from build123d import *

# Parameters (mm, degrees)
SKETCH1_R           = 25.25
SKETCH1_R_2         = 12
BOSS_EXTRUDE1_DEPTH = 6
BOSS_EXTRUDE2_START = -5
SKETCH2_R           = 37
SKETCH2_R_2         = 12
BOSS_EXTRUDE2_DEPTH = 5
SKETCH3_R           = 1.5
CUT_EXTRUDE1_DEPTH  = 53.668776329
CUT_EXTRUDE2_START  = -3
SKETCH4_R           = 3.5
CUT_EXTRUDE2_DEPTH  = 56.668776329
CIRPATTERN1_COUNT   = 3
CHAMFER1_SIZE       = 12
CHAMFER1_SIZE_2     = 6.92820323
CHAMFER2_SIZE       = 2
SKETCH5_R           = 2.1
CUT_EXTRUDE3_DEPTH  = 54.46961768
CIRPATTERN2_COUNT   = 6
FILLET1_R           = 1


with BuildPart() as part:
    # Sketch1 → Boss-Extrude1 (new body)
    with BuildSketch(Plane(origin=(0, 0, 0), x_dir=(1, 0, 0), z_dir=(0, 1, 0))):
        with Locations(Location((0, 0, 0), (0, 0, 270))):
            Circle(SKETCH1_R)
        with Locations(Location((0, 0, 0), (0, 0, 270))):
            Circle(SKETCH1_R_2, mode=Mode.SUBTRACT)
    extrude(amount=BOSS_EXTRUDE1_DEPTH)

    # Sketch2 → Boss-Extrude2 (add)
    with BuildSketch(Plane(origin=(0, 0, 0), x_dir=(1, 0, 0), z_dir=(0, 1, 0)).offset(BOSS_EXTRUDE2_START)):
        with Locations(Location((0, 0, 0), (0, 0, 270))):
            Circle(SKETCH2_R)
        with Locations(Location((0, 0, 0), (0, 0, 270))):
            Circle(SKETCH2_R_2, mode=Mode.SUBTRACT)
    extrude(amount=BOSS_EXTRUDE2_DEPTH)

    # Sketch3 → Cut-Extrude1 (cut, through all)
    with BuildSketch(Plane(origin=(0, 0, 0), x_dir=(1, 0, 0), z_dir=(0, 1, 0))):
        with Locations(Location((0, 32, 0), (0, 0, 270))):
            Circle(SKETCH3_R)
    cut_extrude1 = extrude(amount=-CUT_EXTRUDE1_DEPTH, mode=Mode.SUBTRACT)

    # Sketch4 → Cut-Extrude2 (cut)
    with BuildSketch(Plane(origin=(0, 0, 0), x_dir=(1, 0, 0), z_dir=(0, 1, 0)).offset(CUT_EXTRUDE2_START)):
        with Locations(Location((0, 32, 0), (0, 0, 270))):
            Circle(SKETCH4_R)
    cut_extrude2 = extrude(amount=CUT_EXTRUDE2_DEPTH, mode=Mode.SUBTRACT)

    # CirPattern1: Cut-Extrude1, Cut-Extrude2 ×3 about axis
    cirpattern1_axis = Axis((0, 0, 0), (0, 1, 0))
    add([cut_extrude1.rotate(cirpattern1_axis, i * 360 / CIRPATTERN1_COUNT) for i in range(1, CIRPATTERN1_COUNT)], mode=Mode.SUBTRACT)
    add([cut_extrude2.rotate(cirpattern1_axis, i * 360 / CIRPATTERN1_COUNT) for i in range(1, CIRPATTERN1_COUNT)], mode=Mode.SUBTRACT)

    # Chamfer1
    # the kernel refuses this chamfer: 12, 6.92820323 mm, written as the material it takes off along each edge
    with BuildSketch(Plane(origin=(0, -5, 0), x_dir=(0, 0, 1), z_dir=(-1, 0, 0))) as chamfer1_piece_1:
        Polygon((12, CHAMFER1_SIZE), (12 + CHAMFER1_SIZE_2, 0), (12, 0), align=None)
    revolve(axis=Axis((0, -5, 0), (0, 1, 0)), mode=Mode.SUBTRACT)

    # Chamfer2
    # the kernel refuses this chamfer: 2 mm, written as the material it takes off along each edge
    with BuildSketch(Plane(origin=(0, 0, 0), x_dir=(0, 0, 1), z_dir=(-1, 0, 0))) as chamfer2_piece_1:
        Polygon((37 - CHAMFER2_SIZE, 0), (37, -CHAMFER2_SIZE), (37, 0), align=None)
    revolve(axis=Axis((0, 0, 0), (0, 1, 0)), mode=Mode.SUBTRACT)

    # Sketch5 → Cut-Extrude3 (cut, through all)
    with BuildSketch(Plane(origin=(0, 6, 0), x_dir=(1, 0, 0), z_dir=(0, 1, 0))):
        with Locations(Location((0, 16.5, 0), (0, 0, 270))):
            Circle(SKETCH5_R)
    cut_extrude3 = extrude(amount=-CUT_EXTRUDE3_DEPTH, mode=Mode.SUBTRACT)

    # CirPattern2: Cut-Extrude3 ×6 about axis
    cirpattern2_axis = Axis((0, 0, 0), (0, 1, 0))
    for i in range(1, CIRPATTERN2_COUNT):
        add(cut_extrude3.rotate(cirpattern2_axis, i * 360 / CIRPATTERN2_COUNT), mode=Mode.SUBTRACT)

    # Fillet1
    fillet1_edges = [part.edges().sort_by_distance(p)[0] for p in [
        (0, 6, -12.577350269),
    ]]
    fillet(fillet1_edges, radius=FILLET1_R)


solid = part.part
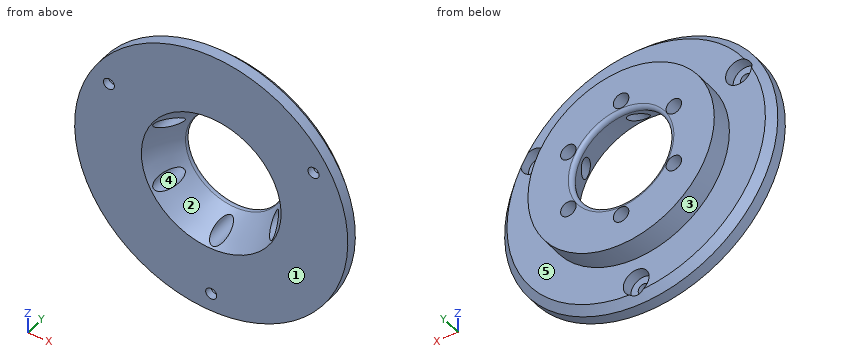
Source: CAD feature listing. Evaluate the final solid. Frame: model axes, mm. Face numbers are marked on the shaded views. A direction names the side the tool comes from. Give positions to 0.01 mm unless a question says otherwise; leave off trailing zeros. Write each loop counter-clockwise with the first axis right and the second up, starting at its lowest first coordinate (ties: lowest second). Pieces come first, ordered by that corner, then holes. Notation, with made-up numbers: (-13.75, -21.5) -> (9.25, -21.5) arc R14 ccw to (9.25, -17.5) -> close; hole circle Ø4 at (43.5, -35.75). An arc over 180 degrees is marked (long way). Write item = value, one per line.
Q1. Line query: line 1 (X direction, y = -4.1, z = 16); line 2 (Y direction, x = -24.5, z = 18.5); line 3 (Z direction, x = 11, y = 4). Output: solid intervals per line, ascending. Write a range as from..to.
Here are the results:
line_1 = -33.36..-29.21, -26.21..-9.1, 9.1..26.21, 29.21..33.36
line_2 = -5..0
line_3 = -22.73..-8.22, 8.22..22.73
Q2. Cut plane A-A on z = 0. Return loops of the section in (x, y), then the cut area to 3 significant figures.
Here are the results:
outline = (-37, -5) -> (-18.93, -5) -> (-13.44, 4.5) arc R1 ccw to (-14.31, 6) -> (-25.25, 6) -> (-25.25, 0) -> (-35, 0) -> (-37, -2) -> close; (13.44, 4.5) -> (18.93, -5) -> (37, -5) -> (37, -2) -> (35, 0) -> (25.25, 0) -> (25.25, 6) -> (14.31, 6) arc R1 ccw to start
area = 321 mm²
Q3. Cut plane B-B on y = 1.75. Return loops of the section in (x, z), then the cut area to 3 significant figures.
Here are the results:
outline = circle Ø50.5 at (0, 0); hole (-13.67, -6.24) arc R2.1 ccw (long way) to (-12.24, -8.72) arc R15.03 ccw to (-1.43, -14.96) arc R2.1 ccw (long way) to (1.43, -14.96) arc R15.03 ccw to (12.24, -8.72) arc R2.1 ccw (long way) to (13.67, -6.24) arc R15.03 ccw to (13.67, 6.24) arc R2.1 ccw (long way) to (12.24, 8.72) arc R15.03 ccw to (1.43, 14.96) arc R2.1 ccw (long way) to (-1.43, 14.96) arc R15.03 ccw to (-12.24, 8.72) arc R2.1 ccw (long way) to (-13.67, 6.24) arc R15.03 ccw to start
area = 1,220 mm²
Q4. Reachability of the marked faces 4 and 5 from +Z, -Z, +X, -X, +Y, -Y: full face, straight path, thin tool, end or side. Return the list, or none.
Here are the results:
face_4 = +Y, -Y
face_5 = +Y
Q5. Mould query, pull axis X, two halves, no side actions, for the marked faces 1, 2 and 3. Classes: +X half, -X half, draft (parallel to the pull), parting line (faces both ways), or undercut.
Here are the results:
face_1 = draft
face_2 = undercut
face_3 = parting line
Q6. First-contact query: pin 1 (2 mm diameter, centred on x = 27.5, z = 14.5, fed in from +Y); pin 2 (4 mm diameter, centred on y = -3, z = -26, fed in from +X); pin 3 (4 mm diameter, centred on x = -17.5, y = -4, fed in from -Z). Flat tips, straight axial feed; report the tip coordinate or a pass-through.
Here are the results:
pin_1 = -3
pin_2 = 28.16
pin_3 = -33.6
Q7. Cut plane C-C on z = 8.25. State how many separate pieces and enclosed holes the cut face has, then the cut area to 3 significant figures.
Here are the results:
separate_pieces = 4
enclosed_holes = 0
area = 290 mm²
